from build123d import *

# Parameters (mm, degrees)
F0_R     = 7.5
F1_DEPTH = 10.668
F5_D     = 2


with BuildPart() as f1:
    # F0 (on Top) → F1 (new body)
    with BuildSketch(Plane.XY):
        Circle(F0_R)
    extrude(amount=F1_DEPTH)

    # F2 (on Right) → F3 (revolve, cut)
    with BuildSketch(Plane.YZ):
        with BuildLine():
            Line((-11.611987, 8.67579), (-11.611987, 7.502463))
            ThreePointArc((-11.611987, 7.502463), (-13.319947, 5.118554), (-11.587891, 2.752094))
            Line((-11.587891, 2.752094), (-11.587891, 1.583694))
            Line((-11.587891, 1.583694), (-2.7, 2.780473))
            Line((-2.7, 2.780473), (-2.7, 7.307734))
            Line((-2.7, 7.307734), (-11.611987, 8.67579))
        make_face()
    revolve(axis=Axis((0, 0, 0), (0, 0, -1)), mode=Mode.SUBTRACT)

    # F5 (through all)
    with Locations(Plane.XY.offset(10.668)):
        with Locations((0, 0)):
            Hole(F5_D / 2)


solid = f1.part
The listing builds one solid part. Answer for the finished solid, in the listing's coordinates (mm). A direction names the side the tool comes from. Round coordinates to 2 decimals unless told otherwise and drop trailing zeros. Write each loop counter-clockwise with the first axis right and the second up, starting at its lowest first coordinate (ties: lowest second). Pieces come first, ordered by that corner, then holes. Notation, with made-up numbers: M 32,-36.5 L 80,-36.5 A33 cw 80,1.5 Z; hole C 85,89.5 d10. An arc over 180 degrees is marked long. Write each question's results on one line, items separated by ' | '. Start each with the question number.
(1) The part is cut by section C-C, the plane z = 9.75. Write down the section's boundary in (x, y), and give its area (3 significant figures).
(2) The part is cut by section A-A, the plane y = 0. Write down the section's boundary in (x, z), and give its area (3 significant figures).
(3) Find the intervals of material crossed by line 1 (Y direction, x = 0, z = 3.5); line 2 (Y direction, x = 0, z = 8.25); line 3 (Z direction, x = 0, y = -4.75), in increasing order.
(4) Each of these flat-tipped pins is pushed along its axis until it touches: P1, Ø2, axis at x = -5.5, z = 9.5, coming from the -Y side; P2, Ø1.5, axis at x = -3.5, z = 8, coming from the +Y side. Where does it stop, or does it pass through?
(5) For faces 4 (the flat face through (2, 0, 0)), 5 (the cylindrical face through (2.636, 0.585, 5.076)), determine the directions among +Z, -Z, +X, -X, +Y, -Y from which every point of the face is accessible in a straight line to the end or side of a thin tool.
(6) Determine the mould class of faces 1 (the cylindrical face through (0, -1, 5)), 2 (the cylindrical face through (-7.493, 0.33, 1.052)), 3 (the flat face through (2, 0, 10.668)) for opening direction X: +X half, -X half, draft (parallel to the pull), parting line (faces both ways), or undercut.
(7) The part is cut by section D-D, the plane z = 2.5. Write down the section's boundary in (x, y), and give its area (3 significant figures).
Worked answers:
1) outline: C 0,0 d15; hole C 0,0 d2 | area: 174 mm²
2) outline: M -7.5,0 L -1,0 L -1,10.67 L -7.5,10.67 L -7.5,8.04 L -2.7,7.31 L -2.7,2.78 L -7.5,2.13 Z; M 1,0 L 7.5,0 L 7.5,2.13 L 2.7,2.78 L 2.7,7.31 L 7.5,8.04 L 7.5,10.67 L 1,10.67 Z | area: 88.6 mm²
3) line 1: y = -2.7 to -1, 1 to 2.7 | line 2: y = -7.5 to -1, 1 to 7.5 | line 3: z = 0 to 2.5, 7.62 to 10.67
4) P1: stops at y = -6 | P2: stops at y = 6.98
5) face 4: -Z, +X, -X, +Y, -Y | face 5: none
6) face 1: undercut | face 2: parting line | face 3: draft
7) outline: C 0,0 d9.57; hole C 0,0 d2 | area: 68.7 mm²
